The model under review builds one solid part; all positions refer to its coordinate system, in mm. A direction names the side the tool comes from. Round coordinates to 2 decimals unless told otherwise and drop trailing zeros. Loops run counter-clockwise (first coordinate to the right, second up) from the corner with the lowest first, then second, coordinate; pieces in that order, holes last. Notation, with made-up numbers: (35.25, 9) -> (83.25, 9) arc R32 cw to (83.25, 40) -> close; hole circle Ø5 at (16, -23.5). An arc over 180 degrees is marked (long way). Write each question's results on one line, items separated by ' | '. Start each with the question number.
Item 1: Mouldability with a two-part tool opening along Z and no side actions: class faces 1 (the flat face through (0.589, 0.599, -1.018)), 2 (the flat face through (27.788, 0, 0)), 3 (the cylindrical face through (2.26, -0.86, 3.88)) as pulls with the +Z half, pulls with the -Z half, needs draft (parallel to the pull), parting line crosses it, or undercut.
Item 2: We need section A-A (z = 0). Give the boundary of the cut face in (x, y).
Item 3: For L1, parallel to X at y = 1.25, z = -3; L2, parallel to X at y = -0.25, z = 0.5; L3, parallel to Z at x = 6.25, y = 0, list the stretches that pass through material, from the lowest coordinate up. Write a range as from..to.
Item 4: Clearance check with flat-ended pins moving along their axes: pin 1 Ø2 at (x, z) = (8, 1) entering from +Y; pin 2 Ø2 at (x, z) = (11, 1.5) entering from +Y; pin 3 Ø1.2 at (y, z) = (0, -0.5) entering from -X. State where each tip first meets the part, or that it passes through.
Item 5: Tool access review of faces 4 (the flat face through (1, -1.181, 0)), 5 (the cylindrical face through (4.284, -0.44, 1.984)), 6 (the flat face through (0, -1.5, 0)), 7 (the cylindrical face through (13.93, -0.52, 2.33)): name each direction out of +Z, -Z, +X, -X, +Y, -Y from which nothing blocks a thin tool from reaching the whole face with its end or side.
Item 6: We need section B-B (x = 15). Give the boundary of the cut face in (y, z), and give its area (3 significant figures).
from build123d import *

# Parameters (mm, degrees)
CUT_EXTRUDE1_DEPTH = 1.1938


# Read off the part's stored shape, not the designer's step: #8-32 Machine Threads Stud1
with BuildPart() as part:
    # Sketch1 → Revolve1 (revolve)
    with BuildSketch(Plane.XY):
        Polygon((0, 0), (0, 3.4671), (0.508, 3.9751), (3.9624, 3.9751), (3.9624, 2.032), (4.5974, 2.032), (4.5974, 2.3876), (23.0124, 2.3876), (23.0124, 1.651), (23.6474, 1.651), (23.6474, 2.0828), (27.7876, 2.0828), (27.7876, 0), align=None)
    revolve(axis=Axis((27.7876, 0, 0), (-1, 0, 0)))

    # #8-32 Machine Threads Stud1 outline → #8-32 Machine Threads Stud1 (revolve, cut)
    with BuildSketch(Plane.YX):
        Polygon((2.0828, 27.7876), (1.61036, 27.7876), (2.0828, 27.31516), align=None)
    revolve(axis=Axis((0, 0, 0), (1, 0, 0)), mode=Mode.SUBTRACT)

    # Sketch3 → Cut-Extrude1 (cut)
    with BuildSketch(Plane.ZY):
        Polygon((1.363816806, 0), (0.681908403, 1.1811), (-0.681908403, 1.1811), (-1.363816806, 0), (-0.681908403, -1.1811), (0.681908403, -1.1811), align=None)
    extrude(amount=-CUT_EXTRUDE1_DEPTH, mode=Mode.SUBTRACT)


solid = part.part
Here are the results:
1) face 1: undercut | face 2: needs draft | face 3: parting line crosses it
2) outline: (0, -3.47) -> (0.51, -3.98) -> (3.96, -3.98) -> (3.96, -2.03) -> (4.6, -2.03) -> (4.6, -2.39) -> (23.01, -2.39) -> (23.01, -1.65) -> (23.65, -1.65) -> (23.65, -2.08) -> (27.32, -2.08) -> (27.79, -1.61) -> (27.79, 1.61) -> (27.32, 2.08) -> (23.65, 2.08) -> (23.65, 1.65) -> (23.01, 1.65) -> (23.01, 2.39) -> (4.6, 2.39) -> (4.6, 2.03) -> (3.96, 2.03) -> (3.96, 3.98) -> (0.51, 3.98) -> (0, 3.47) -> (0, 1.18) -> (1.19, 1.18) -> (1.19, -1.18) -> (0, -1.18) -> close
3) L1: x = 0..3.96 | L2: x = 1.19..27.79 | L3: z = -2.39..2.39
4) pin 1: stops at y = 2.39 | pin 2: stops at y = 2.33 | pin 3: stops at x = 1.19
5) face 4: -X | face 5: none | face 6: +Z, -Z, -X, +Y, -Y | face 7: +X
6) outline: circle Ø4.78 at (0, 0) | area: 17.9 mm2
